Geometry check sheet. Reference: drawing and pictorial views, mm from the part's lowest x, y, z. A direction names the side the tool comes from. Round coordinates to 2 decimals unless told otherwise and drop trailing zeros. Write each loop counter-clockwise with the first axis right and the second up, starting at its lowest first coordinate (ties: lowest second). Pieces come first, ordered by that corner, then holes. Notation, with made-up numbers: M 11,5.5 L 24,5.5 A12 ccw 24,19.5 Z; hole C 71.25,19.5 d1. An arc over 180 degrees is marked long. Answer in a Markdown table with one row per item. Add a question column.
1. Sectioned sample at D-D on y = 10.25. Record the cut outline in (x, z), plus the area to 3 significant figures.
2. Draft check along Z on the marked faces 1, 2 and 3. Enter one of: pulls with the +Z half, pulls with the -Z half, needs draft (parallel to the pull), parting line crosses it, or undercut.
3. Material ranges on probe 1 along Y at (x, z) = (2.2, 28); probe 2 along Z at (x, y) = (2.5, 8); probe 3 along Y at (x, z) = (9.5, 0.55), recorded low to high.
4. Set-up check for the marked faces 4 and 5: record each of +Z, -Z, +X, -X, +Y, -Y from which the full face is reachable in a straight line by a thin tool's end or side.
5. Sectioned sample at C-C on x = 17.75. Record the cut outline in (y, z), plus the area to 3 significant figures.
6. Sectioned sample at A-A on y = 30.25. Record the cut outline in (x, z), plus the area to 3 significant figures.
7. Sectioned sample at B-B on z = 20. Record the cut outline in (x, y).
8. Go/stop test with flat-tipped pins: pin 1 Ø17 at (y, z) = (16, 26) entering from +X; pin 2 Ø8 at (x, z) = (6, 22.5) entering from +Y. Record where each tip stops, or that it passes through.
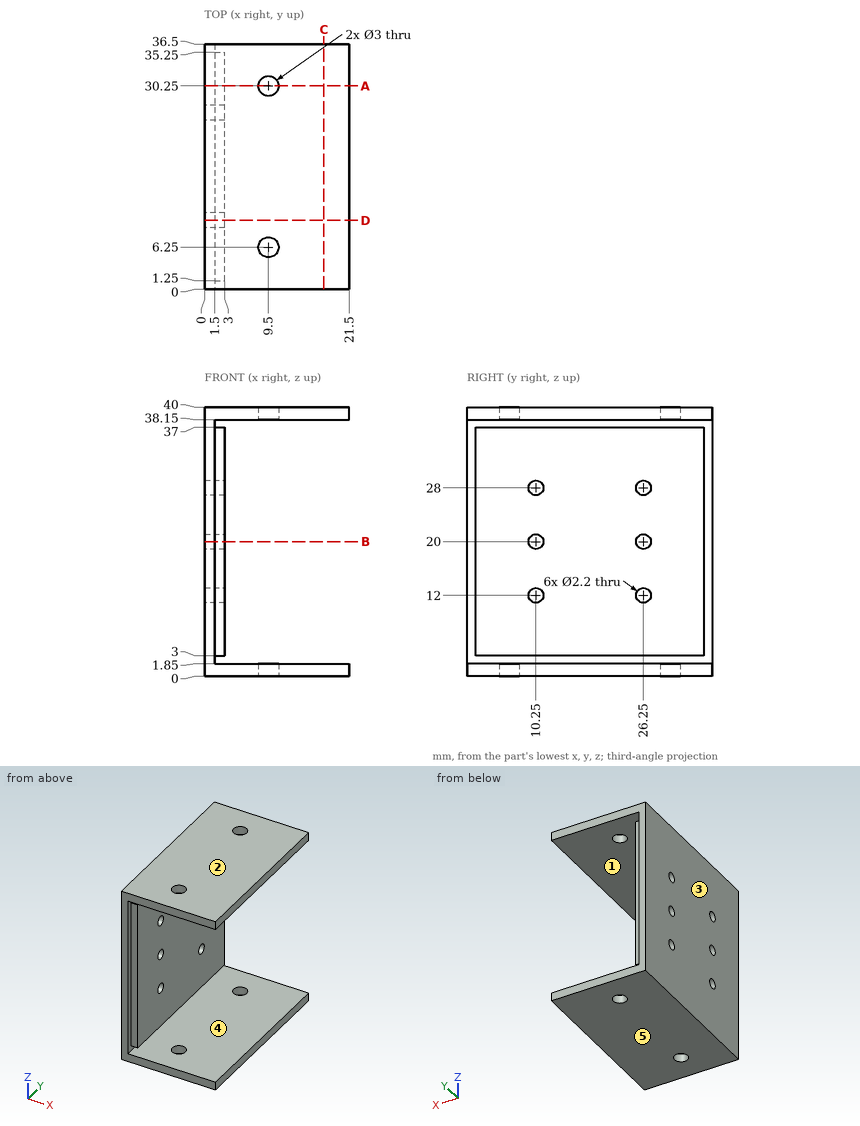
Geometry check:
| question | item | result |
|---|---|---|
| 1 | outline | M 0,0 L 21.5,0 L 21.5,1.85 L 1.5,1.85 L 1.5,3 L 3,3 L 3,10.9 L 0,10.9 Z; M 0,13.1 L 3,13.1 L 3,18.9 L 0,18.9 Z; M 0,21.1 L 3,21.1 L 3,26.9 L 0,26.9 Z; M 0,29.1 L 3,29.1 L 3,37 L 1.5,37 L 1.5,38.15 L 21.5,38.15 L 21.5,40 L 0,40 Z |
| 1 | area | 165 mm2 |
| 2 | face 1 | undercut |
| 2 | face 2 | pulls with the +Z half |
| 2 | face 3 | needs draft |
| 3 | probe 1 | y = 1.25 to 9.15, 11.35 to 25.15, 27.35 to 35.25 |
| 3 | probe 2 | z = 0 to 1.85, 3 to 37, 38.15 to 40 |
| 3 | probe 3 | y = 0 to 4.75, 7.75 to 28.75, 31.75 to 36.5 |
| 4 | face 4 | +X, +Y, -Y |
| 4 | face 5 | -Z, +X, -X, +Y, -Y |
| 5 | outline | M 0,0 L 36.5,0 L 36.5,1.85 L 0,1.85 Z; M 0,38.15 L 36.5,38.15 L 36.5,40 L 0,40 Z |
| 5 | area | 135 mm2 |
| 6 | outline | M 0,0 L 8,0 L 8,1.85 L 1.5,1.85 L 1.5,3 L 3,3 L 3,37 L 1.5,37 L 1.5,38.15 L 8,38.15 L 8,40 L 0,40 Z; M 11,0 L 21.5,0 L 21.5,1.85 L 11,1.85 Z; M 11,38.15 L 21.5,38.15 L 21.5,40 L 11,40 Z |
| 6 | area | 174 mm2 |
| 7 | outline | M 0,0 L 1.5,0 L 1.5,1.25 L 3,1.25 L 3,9.15 L 0,9.15 Z; M 0,11.35 L 3,11.35 L 3,25.15 L 0,25.15 Z; M 0,27.35 L 3,27.35 L 3,35.25 L 1.5,35.25 L 1.5,36.5 L 0,36.5 Z |
| 8 | pin 1 | stops at x = 3 |
| 8 | pin 2 | stops at y = 35.25 |
